Job drawing, mm, ordinate dimensions from the low corner. One solid piece. A direction names the side the tool comes from. Give positions to 0.01 mm unless a question says otherwise; leave off trailing zeros. Order: outer loops, then holes, each group sorted by start corner. A loop starts at its lowest first (then second) coordinate and runs counter-clockwise, first axis right, second up. Notation, with made-up numbers: (80, 60.25) -> (111, 60.25) arc R21 ccw to (111, 95.25) -> close; hole circle Ø8 at (52.5, 53). An arc over 180 degrees is marked (long way). Use CSV: the item, a comma, the result in double quotes. Start each with the question number.
1. Drop a flat-ended pin along its axis: pin 1 (2 mm diameter, centred on x = 5.5, y = 5, fed in from -Z). Give the stop position or say it passes through.
2. Cut at B-B on x = 5. List the corners of the cut face in (y, z) (3 decimals).
3. Cut at A-A on y = 5. List the corners of the cut face in (x, z).
4. Pull direction X, two halves, no side cores. Call the marked faces 3, 4 and 5: released by +X, released by -X, zero draft, split by the parting line, or undercut.
5. 3-axis set-ups, long thin cutter, end or side, ignore diameter. For the marked faces 1 and 2: which of +Z, -Z, +X, -X, +Y, -Y reach the whole face in a straight line?
6. Wall check: line 1 (X direction, y = 8.75, z = 1); line 2 (Y direction, x = 5, z = 12.6); line 3 (Y direction, x = 5.5, z = 1) (3 decimals). Give the ranges that are in metal, low to high. Write a range as from..to.
7. Cut at C-C on z = 10.25. List the corners of the cut face in (x, y) (1 decimal).
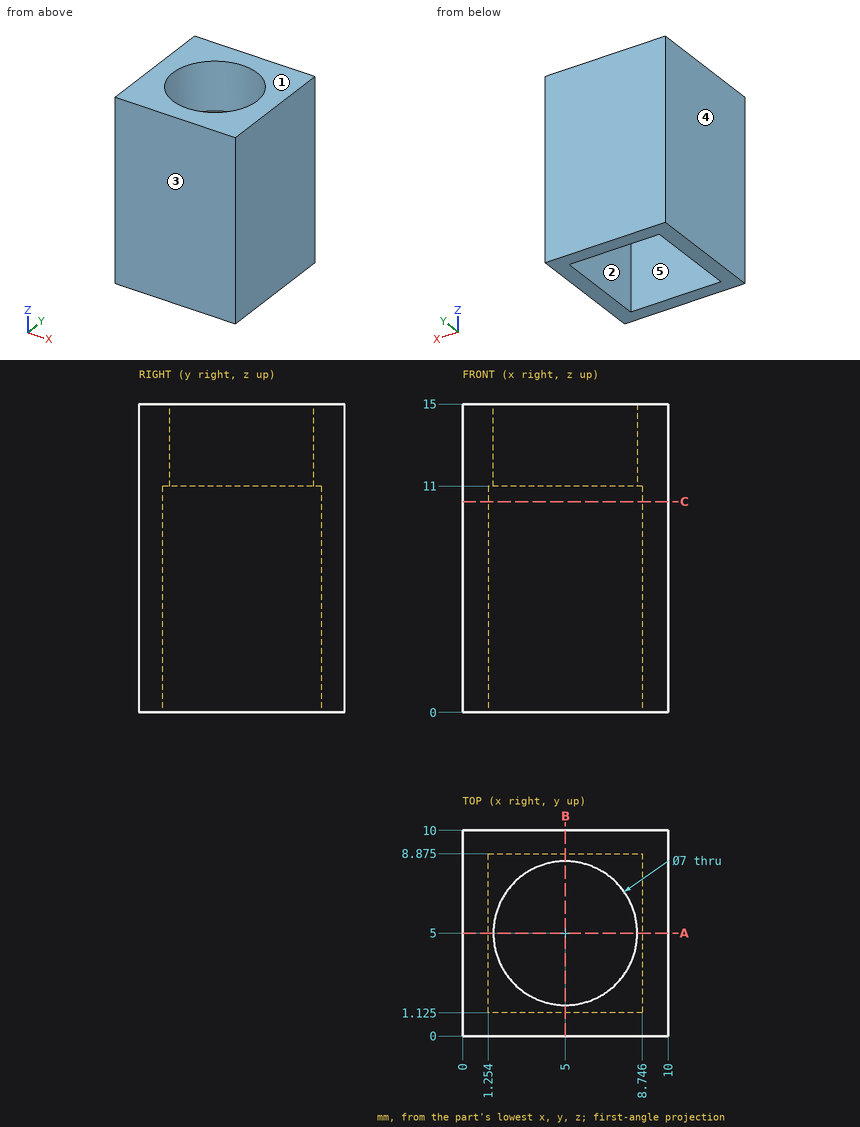
Verdict:
1,pin 1,"through"
2,outline,"(0, 0) -> (1.125, 0) -> (1.125, 11) -> (1.5, 11) -> (1.5, 15) -> (0, 15) -> close; (8.5, 11) -> (8.875, 11) -> (8.875, 0) -> (10, 0) -> (10, 15) -> (8.5, 15) -> close"
3,outline,"(0, 0) -> (1.25, 0) -> (1.25, 11) -> (1.5, 11) -> (1.5, 15) -> (0, 15) -> close; (8.5, 11) -> (8.75, 11) -> (8.75, 0) -> (10, 0) -> (10, 15) -> (8.5, 15) -> close"
4,face 3,"zero draft"
4,face 4,"released by -X"
4,face 5,"undercut"
5,face 1,"+Z, +X, -X, +Y, -Y"
5,face 2,"-Z"
6,line 1,"0..1.25, 8.75..10"
6,line 2,"0..1.5, 8.5..10"
6,line 3,"0..1.125, 8.875..10"
7,outline,"(0, 0) -> (10, 0) -> (10, 10) -> (0, 10) -> close; hole (1.3, 1.1) -> (8.7, 1.1) -> (8.7, 8.9) -> (1.3, 8.9) -> close"
